```python
from build123d import *

# Parameters (mm, degrees)
SKETCH2_R                = 2
BOSS_EXTRUDE1_DEPTH      = 22
BOSS_EXTRUDE2_DEPTH      = 8
BOSS_EXTRUDE2_DEPTH_BACK = 8
SKETCH5_R                = 2
CUT_EXTRUDE1_DEPTH       = 2
CUT_EXTRUDE1_DEPTH_BACK  = 2


with BuildPart() as part:
    # Sketch2 → Boss-Extrude1 (new body)
    with BuildSketch(Plane.YZ):
        with BuildLine():
            Line((14.2713029, 4.10781366), (3.081429665, -3.937612376))
            Line((3.081429665, -3.937612376), (2.751400089, -4.174900903))
            ThreePointArc((2.751400089, -4.174900903), (-2.370970219, -4.402101796), (-5, 0))
            Line((-5, 0), (-5, 57))
            ThreePointArc((-5, 57), (2.726338919, 54.181703922), (6.823492726, 47.050614486))
            Line((6.823492726, 47.050614486), (14.2713029, 4.10781366))
        make_face()
        with Locations(Location((0, 0, 0), (0, 0, 270))):
            Circle(SKETCH2_R, mode=Mode.SUBTRACT)
    extrude(amount=BOSS_EXTRUDE1_DEPTH)

    # Sketch5 → Boss-Extrude2 (add, two sides: drawn at the far end of the back side and taken through both)
    with BuildSketch(Plane.YZ.offset(11).offset(-BOSS_EXTRUDE2_DEPTH_BACK)):
        with BuildLine():
            Line((14.2713029, 4.10781366), (14.983744003, 0))
            Line((14.983744003, 0), (17.876610129, -7.014153205))
            ThreePointArc((17.876610129, -7.014153205), (15.774722197, -11.584740035), (10.865645594, -10.48512021))
            Line((10.865645594, -10.48512021), (4.732907846, -2.750213262))
            Line((4.732907846, -2.750213262), (14.2713029, 4.10781366))
        make_face()
        with Locations(Location((14, -8, 0), (0, 0, 270))):
            Circle(SKETCH5_R, mode=Mode.SUBTRACT)
    extrude(amount=BOSS_EXTRUDE2_DEPTH + BOSS_EXTRUDE2_DEPTH_BACK)

    # Sketch6 → Cut-Extrude1 (cut, two sides: drawn at the far end of the back side and taken through both)
    with BuildSketch(Plane.YZ.offset(11).offset(-CUT_EXTRUDE1_DEPTH_BACK)):
        with BuildLine():
            Line((14.027483372, 5.513635398), (14.4433748, 3.11567649))
            Line((14.4433748, 3.11567649), (14.983744003, 0))
            Line((14.983744003, 0), (17.444478514, -5.966390458))
            ThreePointArc((17.444478514, -5.966390458), (16.264679643, -11.297154245), (10.865645594, -10.48512021))
            Line((10.865645594, -10.48512021), (4.41644607, -2.351076288))
            ThreePointArc((4.41644607, -2.351076288), (8.013457441, 1.376361406), (12.908459217, 3.070834826))
            ThreePointArc((12.908459217, 3.070834826), (13.846657415, 4.118762533), (14.027483372, 5.513635398))
        make_face()
    extrude(amount=CUT_EXTRUDE1_DEPTH + CUT_EXTRUDE1_DEPTH_BACK, mode=Mode.SUBTRACT)


solid = part.part
```
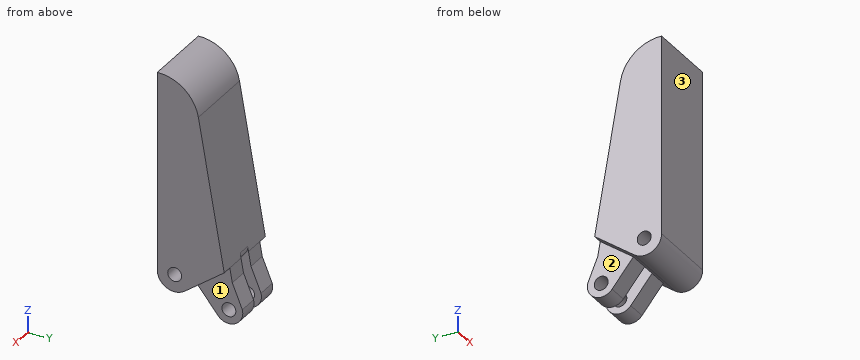
For this review, take the finished solid that the model builds, in its own axes (mm). Face numbers are marked on the shaded views. A direction names the side the tool comes from. Round coordinates to 2 decimals unless told otherwise and drop trailing zeros. Write each loop counter-clockwise with the first axis right and the second up, starting at its lowest first coordinate (ties: lowest second). Pieces come first, ordered by that corner, then holes. Notation, with made-up numbers: (42.5, -25) - (52.5, -25) arc R24 cw to (52.5, -5) - close; hole circle Ø8 at (45, 2.25). An arc over 180 degrees is marked (long way). Put each result on its own line as item: value.
Q1. Wall thickness on probe 1 along Y at (x, z) = (16.25, -8); probe 2 along Y at (x, z) = (7, -4.5); probe 3 along Z at (x, y) = (13.25, -1.25): over which ranges is each line inside the solid? List them lowest first.
Solved:
probe 1: y = 8.9 to 12, 16 to 18
probe 2: y = -2.18 to 2.18, 6.12 to 16.84
probe 3: z = -4.84 to -1.56, 1.56 to 56.4
Q2. Insertion check: pin 1 Ø4 at (x, y) = (5.5, 0) entering from +Z; pin 2 Ø1.5 at (x, y) = (6, 2) entering from -Z; pin 3 Ø8 at (x, y) = (12.5, 8) entering from +Z. Each pin has a flat end and moves straight along its axis. Give the tip position at first contact, or say it passes through.
Solved:
pin 1: stops at z = 56.62
pin 2: stops at z = -4.84
pin 3: stops at z = 52.94
Q3. We need section D-D (y = 0). Give the boundary of the cut face in (x, z), and give its area (3 significant figures).
Solved:
outline: (0, -5) - (22, -5) - (22, -2) - (0, -2) - close; (0, 2) - (22, 2) - (22, 55.91) - (0, 55.91) - close
area: 1,250 mm2
Q4. We need section A-A (x = 14). Give the boundary of the cut face in (y, z).
Solved:
outline: (-5, 0) arc R5 ccw to (2.75, -4.17) - (4.73, -2.75) - (10.87, -10.49) arc R4 ccw to (17.88, -7.01) - (14.98, 0) - (6.82, 47.05) arc R12 ccw to (-5, 57) - close; hole circle Ø4 at (0, 0); hole circle Ø4 at (14, -8)
Q5. Machinability: for the marked faces 1, 2 and 3, which of the approach directions +Z, -Z, +X, -X, +Y, -Y give a long, thin tool a straight path to every point of the face, cutting with its end or side? Answer none if there is none.
Solved:
face 1: -Z, +X, +Y
face 2: -Z, -X, +Y
face 3: +Z, -Z, +X, -X, -Y
Q6. We need section B-B (x = 2). Give the boundary of the cut face in (y, z).
Solved:
outline: (-5, 0) arc R5 ccw to (2.75, -4.17) - (14.27, 4.11) - (6.82, 47.05) arc R12 ccw to (-5, 57) - close; hole circle Ø4 at (0, 0)
Q7. We need section C-C (z = -8). Give the boundary of the cut face in (x, y).
Solved:
outline: (3, 8.9) - (9, 8.9) - (9, 12) - (3, 12) - close; (3, 16) - (9, 16) - (9, 18) - (3, 18) - close; (13, 8.9) - (19, 8.9) - (19, 12) - (13, 12) - close; (13, 16) - (19, 16) - (19, 18) - (13, 18) - close
